Can you work these out from the model? Positions are in its coordinate system, mm. A direction names the side the tool comes from. Coordinates: 2 decimals unless noted, no trailing zeros. Loops run counter-clockwise (first coordinate to the right, second up) from the corner with the lowest first, then second, coordinate; pieces in that order, holes last.
Autodesk Inventor part; units mm, degrees
ref_plane "Work Plane1" through (0, -1.58, 0) normal (1, 0, 0) x (0, 0, 1)
ref_plane "YZ Plane" through (0, 0, 0) normal (1, 0, 0) x (0, 1, 0)
ref_plane "XZ Plane" through (0, 0, 0) normal (0, 1, 0) x (-1, 0, 0)
sketch "草图1" plane through (0, 0, 0) normal (0, 0, 1) x (1, 0, 0)
  arc A0 (2, -34.2689) -> (-2, -34.2689) centre (0, -1.58) ccw
  line L0 (0, 47.3657) -> (0, -51.0943)
  line L1 (-46.62, 0) -> (46.62, 0)
  line L2 (-2, -34.2689) -> (-2, -42.9189)
  line L3 (-2, -6.5402) -> (-2, -13.29) construction
  line L4 (-2.7947, 37.49) -> (3.6722, 37.49) construction
  arc A1 (12.0452, -35.5023) -> (-12.0452, -35.5023) centre (0, 0) ccw
  arc A2 (-9.2384, -41.923) -> (-2, -42.9189) centre (0, -1.58) ccw
  arc A3 (-10, -41.1218) -> (-9.2384, -41.923) centre (-9.0152, -40.9482) ccw
  arc A4 (-10.7182, -37.049) -> (-12.0452, -35.5023) centre (-12.6878, -37.3963) ccw
  line L5 (2, -34.2689) -> (2, -42.9189)
  line L6 (2, -6.5402) -> (2, -13.29) construction
  arc A5 (2, -42.9189) -> (9.2384, -41.923) centre (0, -1.58) ccw
  arc A6 (9.2384, -41.923) -> (10, -41.1218) centre (9.0152, -40.9482) ccw
  circle A7 centre (-6, -38.3943) radius 1.5
  circle A8 centre (6, -38.3943) radius 1.5
  line L7 (-10.7182, -37.049) -> (-10, -41.1218)
  arc A9 (12.0452, -35.5023) -> (10.7182, -37.049) centre (12.6878, -37.3963) ccw
  line L8 (10, -41.1218) -> (10.7182, -37.049)
  arc A10 (-4.8129, -38.5682) -> (5.574, -38.4612) centre (0, -1.58) ccw construction
  dimension "d0" = 65.5
  dimension "d1" = 8.65
  dimension "d6" = 2
  dimension "d8" = 1.58
  dimension "d9" = 1
  dimension "d10" = 2
  dimension "d12" = 3
  dimension "d13" = 3
  dimension "d43" = 10
  dimension "d44" = 37.3
  dimension "d45" = 12
  dimension "d46" = 20
  dimension "d47" = 6.32
extrude "轴承体" add sketch "草图1" along normal blind 2.5 contours A0 L1 A1 A9 L8 A6 A5 L5 | A0 L0 A1 L1 | A0 L1 A1 L0 | A0 L2 A2 A3 L7 A4 A1 L1
ref_plane "Work Plane1" through (0, -1.58, 0) normal (1, 0, 0) x (0, 0, 1)
equation "\"d0\" = ND"
equation "\"d1\" = SRB2"
equation "\"d6\" = 0.5 * B1"
equation "\"d8\" = C1"
equation "\"d9\" = R3"
equation "\"d10\" = R2"
equation "\"d12\" = SD5"
equation "\"d13\" = SD5"
equation "\"d44\" = R1"
equation "\"d45\" = B2"
equation "\"d46\" = L"
equation "\"d47\" = SRB1"
equation "\"d2\" = SD"
equation "\"SD\" = 2.5"
equation "\"SRB1\" = 6.32"
equation "\"ND\" = 65.5"
equation "\"SRB2\" = 8.65"
equation "\"SD5\" = 3"
equation "\"B1\" = 4"
equation "\"R2\" = 2"
equation "\"R3\" = 1"
equation "\"B2\" = 12"
equation "\"R1\" = 37.3"
equation "\"C1\" = 1.58"
equation "\"SD3\" = 65.5"
equation "\"WDMAX\" = 72"
equation "\"H1\" = 0"
properties part number "弹性挡圈GB 894.1-86 - 70" material "钢，软"
Item 1: Suppose I cut it at C-C, the plane z = 1.1. Please give me the cut outline in (x, y).
Results are:
outline: (-12.05, -35.5) arc R2 cw to (-10.72, -37.05) - (-10, -41.12) arc R1 ccw to (-9.24, -41.92) arc R41.39 ccw to (-2, -42.92) - (-2, -34.27) arc R32.75 cw (long way) to (2, -34.27) - (2, -42.92) arc R41.39 ccw to (9.24, -41.92) arc R1 ccw to (10, -41.12) - (10.72, -37.05) arc R2 cw to (12.05, -35.5) arc R37.49 ccw (long way) to start; hole circle Ø3 at (-6, -38.39); hole circle Ø3 at (6, -38.39)
Item 2: Suppose I cut it at D-D, the plane x = -6.5. Please give me the cut outline in (y, z).
Results are:
outline: (-42.45, 0) - (-39.81, 0) - (-39.81, 2.5) - (-42.45, 2.5) - close; (-36.98, 0) - (-33.68, 0) - (-33.68, 2.5) - (-36.98, 2.5) - close; (30.52, 0) - (36.92, 0) - (36.92, 2.5) - (30.52, 2.5) - close
Item 3: On a 3-axis mill with a long thin cutter (end or side, diameter ignored), from which of +Z, -Z, +X, -X, +Y, -Y can I reach the whole of each face in a straight line? I mean faces 1 (the face through (5.692, -42.574, 1.232)), 2 (the face through (2, -39, 1)). Say none if no direction works.
Results are:
face 1: +Z, -Z, +X, -Y
face 2: +Z, -Z, -Y
Item 4: We'd pull the mould along X, two halves only. Please class faces 3 (the face through (-2, -39, 1)), 4 (the face through (-5.59, -42.59, 1.23)), 5 (the face through (-8.51, 30.23, 2.5)): +X half, -X half, draft (parallel to the pull), parting line (faces both ways), or undercut.
Results are:
face 3: undercut
face 4: -X half
face 5: draft
Item 5: I need wall thicknesses on line 1 along Y through (x, z) = (6, 0.65); line 2 along X through (y, z) = (-1.58, 1.65); line 3 along X through (y, z) = (-23, 1.3). Which ranges of each line are inside material? Lowest first, please.
Results are:
line 1: y = -42.53 to -39.89, -36.89 to -33.78, 30.62 to 37.01
line 2: x = -37.46 to -32.75, 32.75 to 37.46
line 3: x = -29.61 to -24.77, 24.77 to 29.61
Item 6: Suppose I cut it at A-A, the plane x = -14. Please give me the cut outline in (y, z).
Results are:
outline: (-34.78, 0) - (-31.19, 0) - (-31.19, 2.5) - (-34.78, 2.5) - close; (28.03, 0) - (34.78, 0) - (34.78, 2.5) - (28.03, 2.5) - close
Item 7: Suppose I cut it at B-B, the plane y = -1. Please give me the cut outline in (x, z), plus the area to 3 significant figures.
Results are:
outline: (-37.48, 0) - (-32.74, 0) - (-32.74, 2.5) - (-37.48, 2.5) - close; (32.74, 0) - (37.48, 0) - (37.48, 2.5) - (32.74, 2.5) - close
area: 23.7 mm2
Item 8: I'm going to push flat-ended pins straight in: P1, Ø1.5, axis at y = -15, z = 1.5, coming from the +X side; P2, Ø0.8, axis at y = -37.5, z = 1.5, coming from the -X side; P3, Ø1.2, axis at y = -39, z = 1, coming from the +X side. Where does each tip first touch, or does it pass through?
Results are:
P1: stops at x = 34.68
P2: stops at x = -10.71
P3: stops at x = 10.48
